Geometry: final body of the model. Coordinates: model frame, mm. Face numbers are marked on the shaded views. A direction names the side the tool comes from. Round coordinates to 2 decimals unless told otherwise and drop trailing zeros. Write each loop counter-clockwise with the first axis right and the second up, starting at its lowest first coordinate (ties: lowest second). Pieces come first, ordered by that corner, then holes. Notation, with made-up numbers: (-31.5, -29.75) - (6.5, -29.75) arc R17 cw to (6.5, -22.75) - close; hole circle Ø3 at (-16, 62.5). An arc over 180 degrees is marked (long way). Write each question's results on one line, items separated by ' | '.
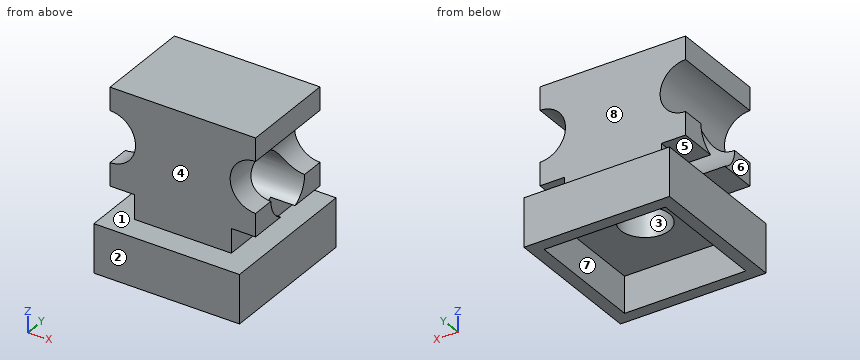
Autodesk Fusion 360 part; units mm, degrees
sketch "草图1" plane through (0, 0, 0) normal (0, 0, 1) x (1, 0, 0)
  line L0 (0, 10) -> (6, 10)
  line L1 (6, 10) -> (6, 3.9983)
  line L2 (6, 3.9983) -> (0, 3.9983)
  line L3 (0, 3.9983) -> (0, 10)
  dimension "d1" = 6
extrude "拉伸1" add sketch "草图1" along normal blind 2
sketch "草图2" plane through (0, 0, 0) normal (0, 0, -1) x (1, 0, 0)
  line L0 (6, -3.9983) -> (0, -3.9983)
  line L1 (0, -3.9983) -> (0, -10)
  line L2 (0, -10) -> (6, -10)
  line L3 (6, -10) -> (6, -3.9983)
sketch "草图3" plane through (0, 0, 0) normal (0, 0, -1) x (1, 0, 0)
  line L0 (5.5, -9.5) -> (0.5, -9.5)
  line L1 (0.5, -9.5) -> (0.5, -4.5)
  line L2 (0.5, -4.5) -> (5.5, -4.5)
  line L3 (5.5, -4.5) -> (5.5, -9.5)
extrude "拉伸2" cut sketch "草图3" against normal blind 1.5
sketch "草图4" plane through (0, 0, 2) normal (0, 0, 1) x (-1, 0, 0)
  line L0 (0, -3.9983) -> (-6, -3.9983)
  line L1 (-6, -3.9983) -> (-6, -10)
  line L2 (-6, -10) -> (0, -10)
  line L3 (0, -10) -> (0, -3.9983)
  line L4 (-5, -5) -> (-1, -5)
  line L5 (-1, -5) -> (-1, -9)
  line L6 (-1, -9) -> (-5, -9)
  line L7 (-5, -9) -> (-5, -5)
extrude "拉伸3" add sketch "草图4" along normal blind 1 contours L4 L5 L6 L7
sketch "草图5" plane through (0, 0, 3) normal (0, 0, 1) x (-1, 0, 0)
  line L0 (-5, -9) -> (-1, -9)
  line L1 (-1, -9) -> (-1, -5)
  line L2 (-1, -5) -> (-5, -5)
  line L3 (-5, -5) -> (-5, -9)
  line L4 (-6, -5) -> (0, -5)
  line L5 (0, -5) -> (0, -9)
  line L6 (0, -9) -> (-6, -9)
  line L7 (-6, -9) -> (-6, -5)
extrude "拉伸4" add sketch "草图5" along normal blind 4
hole "孔1" at (6, 9, 5) direction (0, -1, 0) diameter 2.1 depth 6.5 tip angle 118
hole "孔2" at (0, 9, 5) direction (0, -1, 0) diameter 2.1 depth 6.5 tip angle 118
hole "孔3" at (0, 7, 3.95) direction (1, 0, 0) diameter 2.1 depth 6.5 tip angle 118
sketch "草图6" plane through (0, 0, 7) normal (0, 0, 1) x (-1, 0, 0)
  line L0 (-6, -9) -> (0, -9)
  line L1 (0, -9) -> (0, -5)
  line L2 (0, -5) -> (-6, -5)
  line L3 (-6, -5) -> (-6, -9)
hole "孔4" at (2.9657, 7.0441, 1.5) direction (0, 0, 1) diameter 2 depth 4 tip angle 118
Q1. Access query for the marked faces 4, 5, 6, 7 and 8. Directions: +Z, -Z, +X, -X, +Y, -Y. A direction counts if a zero-diameter tool reaches every point of the face in a straight line with its end or side. Return the directions, or none.
Answer block:
face 4: +Z, +X, -X, -Y | face 5: -X, +Y, -Y | face 6: +Z, -Z, -X, +Y, -Y | face 7: -Z | face 8: +Z, +X, -X, +Y
Q2. Ray query, line 1 along Y through (x, z) = (2, 4); line 2 along X through (y, z) = (7, 0.5); line 3 along Z through (x, y) = (5.75, 6.25). Return the intervals inside material, ascending.
Answer block:
line 1: 5 to 5.95, 8.05 to 9 | line 2: 0 to 0.5, 5.5 to 6 | line 3: 0 to 2, 3 to 3.22, 6.02 to 7
Q3. Mould query, pull axis Y, two halves, no side actions, for the marked faces 1, 2 and 3. Classes: pulls with the +Y half, pulls with the -Y half, needs draft (parallel to the pull), parting line crosses it, or undercut.
Answer block:
face 1: needs draft | face 2: pulls with the -Y half | face 3: undercut
Q4. Section query C-C, the plane z = 1.25. Return loops of the section in (x, y).
Answer block:
outline: (0, 4) - (6, 4) - (6, 10) - (0, 10) - close; hole (0.5, 4.5) - (5.5, 4.5) - (5.5, 9.5) - (0.5, 9.5) - close
Q5. Section query B-B, the plane z = 4.25. Return loops of the section in (x, y).
Answer block:
outline: (0.73, 5) - (5.27, 5) - (5.27, 5.99) - (0.73, 5.99) - close; (0.73, 8.01) - (2.69, 8.01) arc R1 cw to (3.24, 8.01) - (5.27, 8.01) - (5.27, 9) - (0.73, 9) - close
Q6. Pin query (flat end, axial travel): pin 1 (1.5 mm diameter, centred on x = 4.5, z = 6, fed in from -Y). Return the tip coordinate at first contact, or that it passes through.
Answer block:
pin 1: y = 5
Q7. Section query A-A, the plane x = 4.75. Return loops of the section in (y, z).
Answer block:
outline: (4, 0) - (4.5, 0) - (4.5, 1.5) - (9.5, 1.5) - (9.5, 0) - (10, 0) - (10, 2) - (9, 2) - (9, 7) - (5, 7) - (5, 2) - (4, 2) - close; hole circle Ø2.1 at (7, 3.95)
Q8. Section query D-D, the plane y = 7.25. Give the number of separate pieces and of enclosed holes in the cut face, plus the area to 3 significant figures.
Answer block:
separate pieces: 3 | enclosed holes: 0 | area: 14.2 mm2
